Verification items for the finished model (mm, model axes). A direction names the side the tool comes from. Give positions to 0.01 mm unless a question says otherwise; leave off trailing zeros. Order: outer loops, then holes, each group sorted by start corner. A loop starts at its lowest first (then second) coordinate and runs counter-clockwise, first axis right, second up. Notation, with made-up numbers: M 40,35.25 L 46,35.25 A16 cw 46,60.25 Z; hole C 58.25,-32 d6. An arc over 180 degrees is marked long. Answer as a JSON object with one key per item and string values.
```python
from build123d import *

# Parameters (mm, degrees)
SKETCH1_W           = 53.5
SKETCH1_H           = 60
SKETCH1_W_2         = 45.5
SKETCH1_H_2         = 52
BOSS_EXTRUDE1_DEPTH = 82
CUT_EXTRUDE1_START  = -4
CUT_EXTRUDE1_DEPTH  = 107.40239255
LPATTERN1_COUNT     = 2
LPATTERN1_PITCH     = 29
CUT_EXTRUDE2_DEPTH  = 4
LPATTERN2_COUNT     = 2
LPATTERN2_PITCH     = 29
BOSS_EXTRUDE2_DEPTH = 53.5
FILLET1_R           = 10
FILLET2_R           = 3
SKETCH6_R           = 1.5
CUT_EXTRUDE3_DEPTH  = 9
CUT_EXTRUDE4_DEPTH  = 105.634635656
CUT_EXTRUDE5_DEPTH  = 110.161184183


with BuildPart() as part:
    # Sketch1 → Boss-Extrude1 (new body)
    with BuildSketch(Plane(origin=(0, 0, 0), x_dir=(1, 0, 0), z_dir=(0, 1, 0))):
        Rectangle(SKETCH1_W, SKETCH1_H)
        Rectangle(SKETCH1_W_2, SKETCH1_H_2, mode=Mode.SUBTRACT)
    extrude(amount=BOSS_EXTRUDE1_DEPTH)

    # Sketch3 → Cut-Extrude1 (cut)
    with BuildSketch(Plane.ZY.offset(26.75).offset(CUT_EXTRUDE1_START)):
        with BuildLine():
            Line((19.5, 76), (19.5, 50))
            ThreePointArc((19.5, 50), (18, 48.5), (16.5, 50))
            Line((16.5, 50), (16.5, 76))
            ThreePointArc((16.5, 76), (18, 77.5), (19.5, 76))
        make_face()
        with BuildLine():
            Line((12.5, 70), (12.5, 42))
            ThreePointArc((12.5, 42), (11, 40.5), (9.5, 42))
            Line((9.5, 42), (9.5, 70))
            ThreePointArc((9.5, 70), (11, 71.5), (12.5, 70))
        make_face()
    cut_extrude1 = extrude(amount=CUT_EXTRUDE1_DEPTH, mode=Mode.SUBTRACT)

    # LPattern1: Cut-Extrude1 ×2
    with Locations(*[(0, 0, -i * LPATTERN1_PITCH) for i in range(1, LPATTERN1_COUNT)]):
        add(cut_extrude1, mode=Mode.SUBTRACT)

    # Sketch4 → Cut-Extrude2 (cut)
    with BuildSketch(Plane(origin=(26.75, 0, 0), x_dir=(0, 0, -1), z_dir=(1, 0, 0))):
        with BuildLine():
            Line((-9.5, 76), (-9.5, 45))
            ThreePointArc((-9.5, 45), (-11, 43.5), (-12.5, 45))
            Line((-12.5, 45), (-12.5, 76))
            ThreePointArc((-12.5, 76), (-11, 77.5), (-9.5, 76))
        make_face()
        with BuildLine():
            Line((-16.5, 70), (-16.5, 42))
            ThreePointArc((-16.5, 42), (-18, 40.5), (-19.5, 42))
            Line((-19.5, 42), (-19.5, 70))
            ThreePointArc((-19.5, 70), (-18, 71.5), (-16.5, 70))
        make_face()
    cut_extrude2 = extrude(amount=-CUT_EXTRUDE2_DEPTH, mode=Mode.SUBTRACT)

    # LPattern2: Cut-Extrude2 ×2
    with Locations(*[(0, 0, -i * LPATTERN2_PITCH) for i in range(1, LPATTERN2_COUNT)]):
        add(cut_extrude2, mode=Mode.SUBTRACT)

    # Sketch5 → Boss-Extrude2 (add, through all)
    with BuildSketch(Plane.ZY.offset(26.75)):
        Polygon((30, 82), (30, 69), (40, 82), align=None)
        Polygon((-30, 82), (-30, 69), (-40, 82), align=None)
    extrude(amount=-BOSS_EXTRUDE2_DEPTH)

    # Fillet1
    fillet1_edges = [part.edges().sort_by_distance(p)[0] for p in [
        (0, 69, 30),
        (0, 69, -30),
    ]]
    fillet(fillet1_edges, radius=FILLET1_R)

    # Fillet2
    fillet2_edges = [part.edges().sort_by_distance(p)[0] for p in [
        (-26.75, 82, 0),
        (0, 82, 40),
        (0, 82, -40),
        (26.75, 76.847944071, -36.036880054),
        (-26.75, 76.847944071, -36.036880054),
        (26.75, 32.799390267, 30),
        (-26.75, 32.799390267, 30),
        (-26.75, 76.847944071, 36.036880054),
        (26.75, 76.847944071, 36.036880054),
        (26.75, 32.799390267, -30),
        (-26.75, 32.799390267, -30),
        (-26.75, 68.818842729, 30.532624468),
        (26.75, 68.818842729, 30.532624468),
        (-26.75, 68.818842729, -30.532624468),
        (26.75, 68.818842729, -30.532624468),
        (26.75, 82, 0),
    ]]
    fillet(fillet2_edges, radius=FILLET2_R)

    # Sketch6 → Cut-Extrude3 (cut)
    with BuildSketch(Plane(origin=(0, 82, 0), x_dir=(1, 0, 0), z_dir=(0, 1, 0))):
        with Locations(Location((-15.75, -30, 0), (0, 0, 270))):
            Circle(SKETCH6_R)
        with Locations(Location((15.75, -30, 0), (0, 0, 90))):
            Circle(SKETCH6_R)
    cut_extrude3 = extrude(amount=-CUT_EXTRUDE3_DEPTH, mode=Mode.SUBTRACT)

    # Mirror1: Cut-Extrude3 across plane
    add(cut_extrude3.mirror(Plane.XY), mode=Mode.SUBTRACT)

    # Sketch7 → Cut-Extrude4 (cut, through all)
    with BuildSketch(Plane(origin=(26.75, 0, 0), x_dir=(0, 0, -1), z_dir=(1, 0, 0))):
        with BuildLine():
            Line((7, 0), (7, 6))
            ThreePointArc((7, 6), (0, 13), (-7, 6))
            Line((-7, 6), (-7, 0))
            Line((-7, 0), (7, 0))
        make_face()
    extrude(amount=-CUT_EXTRUDE4_DEPTH, mode=Mode.SUBTRACT)

    # Sketch8 → Cut-Extrude5 (cut, through all)
    with BuildSketch(Plane(origin=(0, 0, -30), x_dir=(-1, 0, 0), z_dir=(0, 0, -1))):
        with BuildLine():
            Line((7, 0), (7, 6))
            ThreePointArc((7, 6), (0, 13), (-7, 6))
            Line((-7, 6), (-7, 0))
            Line((-7, 0), (7, 0))
        make_face()
    extrude(amount=-CUT_EXTRUDE5_DEPTH, mode=Mode.SUBTRACT)


solid = part.part
```
Q1. Tool access check on faces 4 (the face through (24.8, 77.5, -18)), 5 (the face through (22.75, 40, 0)), 6 (the face through (-24.7, 40.5, -18)). Record the directions out of +Z, -Z, +X, -X, +Y, -Y that give a thin tool (end or side, any length) a straight path to the whole face; none if there is none.
Resolved:
{"face 4": "+X", "face 5": "+Y, -Y", "face 6": "-X"}
Q2. Gauge pin test, flat ends, axial feed: pin 1 Ø3 at (x, y) = (-24, 58.5) entering from -Z; pin 2 Ø0.9 at (x, z) = (-15.5, -30.5) entering from +Y; pin 3 Ø4.5 at (x, y) = (24, 60) entering from +Z. Record the tip position at first contact, or that the pin passes through.
Resolved:
{"pin 1": "stops at z = -30", "pin 2": "stops at y = 73", "pin 3": "stops at z = 30"}
Q3. Material ranges on L1, parallel to X at y = 77, z = 30; L2, parallel to Z at x = 15.75, y = 79.25; L3, parallel to X at y = 41.5, z = -22, recorded low to high.
Resolved:
{"L1": "x = -26.75 to -17.25, -14.25 to 14.25, 17.25 to 26.75", "L2": "z = -36.9 to -31.5, -28.5 to -26, 26 to 28.5, 31.5 to 36.9", "L3": "x = -26.75 to -22.75, 22.75 to 26.75"}
Q4. Section check C-C on z = -18. Record the cut outline in (x, y).
Resolved:
{"outline": "M -26.75,0 L -22.75,0 L -22.75,40.5 L -26.75,40.5 Z; M -26.75,71.5 L -22.75,71.5 L -22.75,82 L -23.75,82 A3 ccw -26.75,79 Z; M 22.75,0 L 26.75,0 L 26.75,43.5 L 22.75,43.5 Z; M 22.75,77.5 L 26.75,77.5 L 26.75,79 A3 ccw 23.75,82 L 22.75,82 Z"}
Q5. Section check D-D on y = 23.5. Record the cut outline in (x, z).
Resolved:
{"outline": "M -26.75,-27 A3 ccw -23.75,-30 L 23.75,-30 A3 ccw 26.75,-27 L 26.75,27 A3 ccw 23.75,30 L -23.75,30 A3 ccw -26.75,27 Z; hole M -22.75,-26 L 22.75,-26 L 22.75,26 L -22.75,26 Z"}
Q6. Section check A-A on z = 21.5. Record the cut outline in (x, y).
Resolved:
{"outline": "M -26.75,0 L -22.75,0 L -22.75,82 L -23.75,82 A3 ccw -26.75,79 Z; M 22.75,0 L 26.75,0 L 26.75,79 A3 ccw 23.75,82 L 22.75,82 Z"}
Q7. Release check for a two-part mould opening along X. For faces 1 (the face through (-7, 3, -28)), 2 (the face through (-24.7, 48.5, -11)), 3 (the face through (-25.89, 33.26, 29.1)) record: +X half, -X half, draft (parallel to the pull), parting line (faces both ways), or undercut.
Resolved:
{"face 1": "undercut", "face 2": "draft", "face 3": "-X half"}
Q8. Section check B-B on x = -15.75. Record the cut outline in (y, z), then the cut area to 3 significant figures.
Resolved:
{"outline": "M 0,-30 L 65.6,-30 A10 cw 71.7,-32.07 L 77.17,-36.29 A3 ccw 82,-33.91 L 82,-31.5 L 73,-31.5 L 73,-28.5 L 82,-28.5 L 82,-26 L 0,-26 Z; M 0,26 L 82,26 L 82,28.5 L 73,28.5 L 73,31.5 L 82,31.5 L 82,33.91 A3 ccw 77.17,36.29 L 71.7,32.07 A10 cw 65.6,30 L 0,30 Z", "area": "718 mm²"}
